```python
from build123d import *

# Parameters (mm, degrees)
SKETCH1_W              = 139.7
SKETCH1_H              = 82.55
BOSS_EXTRUDE1_DEPTH    = 12
F_10_CLEARANCE_HOLE1_D = 5.1054


with BuildPart() as part:
    # Sketch1 → Boss-Extrude1 (new body)
    with BuildSketch(Plane(origin=(0, 0, 0), x_dir=(1, 0, 0), z_dir=(0, 1, 0))):
        Rectangle(SKETCH1_W, SKETCH1_H)
    extrude(amount=BOSS_EXTRUDE1_DEPTH)

    # #10 Clearance Hole1 (through all)
    with Locations(Plane(origin=(0, 0, 0), x_dir=(-1, 0, 0), z_dir=(0, -1, 0))):
        with Locations((-50.8, 25.781), (0, 25.781), (50.8, 25.781), (50.8, -25.781), (0, -25.781), (-50.8, -25.781)):
            Hole(F_10_CLEARANCE_HOLE1_D / 2)


solid = part.part
```
Geometry: final body of the model. Coordinates: model frame, mm. Coordinates: 2 decimals unless noted, no trailing zeros. Write each loop counter-clockwise with the first axis right and the second up, starting at its lowest first coordinate (ties: lowest second). Pieces come first, ordered by that corner, then holes. Notation, with made-up numbers: M 60,5.25 L 99,5.25 A19 cw 99,33.25 Z; hole C 56.5,78 d2. An arc over 180 degrees is marked long. Use CSV: the item, a comma, the result in double quotes. Start each with the question number.
1. Mould query, pull axis X, two halves, no side actions, for faces 1 (the face through (-0.6, 6.1, -23.3)), 2 (the face through (69.85, 6, 1)), 3 (the face through (-69.85, 6, 1)). Classes: pulls with the +X half, pulls with the -X half, needs draft (parallel to the pull), parting line crosses it, or undercut.
2. First-contact query: P1, Ø6, axis at x = 0, z = -25.781, coming from the -Y side; P2, Ø4, axis at x = -50.8, z = -25.781, coming from the -Y side. Flat tips, straight axial feed; report the tip coordinate or a pass-through.
3. Cut plane A-A on x = 50.8. Return the cut outline in (y, z) (3 decimals), plus the area to 3 significant figures.
4. Ray query, probe 1 along X at (y, z) = (6, 26); probe 2 along Z at (x, y) = (50.8, 3.5) (3 decimals); probe 3 along Z at (x, y) = (48.5, 10.5) (3 decimals). Return the intervals inside material, ascending.
Entries:
1,face 1,"undercut"
1,face 2,"pulls with the +X half"
1,face 3,"pulls with the -X half"
2,P1,"y = 0"
2,P2,"through"
3,outline,"M 0,-41.275 L 12,-41.275 L 12,-28.334 L 0,-28.334 Z; M 0,-23.228 L 12,-23.228 L 12,23.228 L 0,23.228 Z; M 0,28.334 L 12,28.334 L 12,41.275 L 0,41.275 Z"
3,area,"868 mm²"
4,probe 1,"-69.85 to -53.34, -48.26 to -2.54, 2.54 to 48.26, 53.34 to 69.85"
4,probe 2,"-41.275 to -28.334, -23.228 to 23.228, 28.334 to 41.275"
4,probe 3,"-41.275 to -26.888, -24.674 to 24.674, 26.888 to 41.275"
